Autodesk Inventor part; units mm, degrees
ref_plane "YZ Plane" through (0, 0, 0) normal (1, 0, 0) x (0, 1, 0)
ref_plane "XZ Plane" through (0, 0, 0) normal (0, 1, 0) x (-1, 0, 0)
ref_plane "XY Plane" through (0, 0, 0) normal (0, 0, 1) x (1, 0, 0)
sketch "Wireframe" plane through (0, 0, 0) normal (0, 0, 1) x (1, 0, 0)
  line L0 (0, 0) -> (1080, 0)
  line L1 (1080, 0) -> (1080, 750)
  line L2 (1080, 750) -> (0, 750)
  line L3 (0, 750) -> (0, 0)
  dimension "d0" = 1080
  dimension "d1" = 750
extrude "Extrusion1" add sketch "Wireframe" along normal blind 250
sketch "Sketch4" plane through (1080, 0, 0) normal (1, 0, 0) x (0, 0, -1)
  line L0 (0, 0) -> (0, 750)
  line L1 (0, 0) -> (0, 149.657)
  line L2 (0, 0) -> (0, 105)
  line L3 (0, 0) -> (105, 0) construction
  line L4 (0, 105) -> (-100, 105)
  line L5 (-100, 105) -> (-100, 295)
  line L6 (-100, 295) -> (0, 295)
  line L7 (0, 295) -> (0, 455)
  line L8 (0, 455) -> (-100, 455)
  line L9 (-100, 455) -> (-100, 645)
  line L10 (-100, 645) -> (0, 645)
  line L11 (0, 645) -> (0, 750)
  dimension "d8" = 105
  dimension "d9" = 90
  dimension "d10" = 100
  dimension "d11" = 190
  dimension "d12" = 100
  dimension "d13" = 160
  dimension "d14" = 100
  dimension "d15" = 190
  dimension "d16" = 100
extrude "Extrusion2" cut sketch "Sketch4" against normal up to next contours L8 L9 L10 L0
sketch "Sketch5" plane through (1080, 0, 250) normal (1, 0, 0) x (0, 0, -1)
  line L0 (250, 0) -> (250, 105)
  line L1 (250, 0) -> (250, 455)
  line L2 (250, 105) -> (150, 105)
  line L3 (150, 105) -> (150, 295)
  line L4 (150, 295) -> (250, 295)
  dimension "d19" = 105
  dimension "d20" = 100
  dimension "d21" = 190
  dimension "d22" = 100
extrude "Extrusion3" cut sketch "Sketch5" against normal up to next
properties part number "GraniteEpoxyBase" material "Concrete"
Geometry: final body of the model. Coordinates: model frame, mm. A direction names the side the tool comes from. Round coordinates to 2 decimals unless told otherwise and drop trailing zeros. Loops run counter-clockwise (first coordinate to the right, second up) from the corner with the lowest first, then second, coordinate; pieces in that order, holes last. Notation, with made-up numbers: (45.25, -5) -> (50.25, -5) arc R19 ccw to (50.25, 18) -> close; hole circle Ø7 at (65, 16). An arc over 180 degrees is marked (long way). Write each question's results on one line, items separated by ' | '.
Item 1: Pin query (flat end, axial travel): pin 1 Ø3 at (x, y) = (192.5, 577) entering from -Z. Return the tip coordinate at first contact, or that it passes through.
Answers below:
pin 1: stops at z = 100
Item 2: Line query: probe 1 along Y at (x, z) = (700.5, 14); probe 2 along Z at (x, y) = (932, 567.5). Output: solid intervals per line, ascending. Write a range as [from, to].
Answers below:
probe 1: y = [0, 105], [295, 455], [645, 750] | probe 2: z = [100, 250]
Item 3: Cut plane B-B on x = 996.5. Return the cut outline in (y, z), and give its area (4 significant figures).
Answers below:
outline: (0, 0) -> (105, 0) -> (105, 100) -> (295, 100) -> (295, 0) -> (455, 0) -> (455, 100) -> (645, 100) -> (645, 0) -> (750, 0) -> (750, 250) -> (0, 250) -> close | area: 149,500 mm²
Item 4: Set-up query: faces 4 (the face through (532, 380, 250)), 5 (the face through (548, 199, 100)). Return all of +Z, -Z, +X, -X, +Y, -Y with unobstructed straight access to the full face (end or side cutting, diameter ignored); none if empty.
Answers below:
face 4: +Z, +X, -X, +Y, -Y | face 5: -Z, +X, -X
Item 5: Cut plane C-C on y = 609.5. Return the cut outline in (x, z), and give its area (3 significant figures).
Answers below:
outline: (0, 100) -> (1080, 100) -> (1080, 250) -> (0, 250) -> close | area: 162,000 mm²
Item 6: Pull-direction query (Y, two-part tool) for faces 1 (the face through (548, 750, 123)), 2 (the face through (548, 645, 51)), 3 (the face through (532, 376, 0)); classes: pulls with the +Y half, pulls with the -Y half, needs draft (parallel to the pull), parting line crosses it, or undercut.
Answers below:
face 1: pulls with the +Y half | face 2: undercut | face 3: needs draft
Item 7: Cut plane A-A on z = 86.5. Return the cut outline in (x, y).
Answers below:
outline: (0, 0) -> (1080, 0) -> (1080, 105) -> (0, 105) -> close; (0, 295) -> (1080, 295) -> (1080, 455) -> (0, 455) -> close; (0, 645) -> (1080, 645) -> (1080, 750) -> (0, 750) -> close
